Autodesk Inventor part; units mm, degrees
ref_plane "YZ Plane" through (0, 0, 0) normal (1, 0, 0) x (0, 1, 0)
ref_plane "XZ Plane" through (0, 0, 0) normal (0, 1, 0) x (-1, 0, 0)
ref_plane "XY Plane" through (0, 0, 0) normal (0, 0, 1) x (1, 0, 0)
sketch "Sketch1" plane through (0, 0, 0) normal (0, 0, 1) x (1, 0, 0)
  line L0 (-15.9912, -11.7475) -> (15.7588, -11.7475)
  line L1 (15.7588, -11.7475) -> (15.7588, 14.2875)
  line L2 (-15.9912, 14.2875) -> (-15.9912, -11.7475)
  line L3 (-15.9912, -11.7475) -> (15.7588, 11.5768) construction
  line L4 (15.7588, -11.7475) -> (-15.9912, 11.9207) construction
  line L5 (19.1662, -14.2875) -> (-19.1662, -14.2875)
  line L6 (-19.1662, -14.2875) -> (-19.1662, 14.2875)
  line L7 (19.1662, 14.2875) -> (19.1662, -14.2875)
  line L8 (19.1662, -14.2875) -> (-19.1662, 14.2875) construction
  line L9 (-19.1662, -14.2875) -> (19.1662, 14.2875) construction
  line L10 (-19.1662, 14.2875) -> (-15.9912, 14.2875)
  line L11 (15.7588, 14.2875) -> (19.1662, 14.2875)
  point P0 (0, 0)
  dimension "d2" = 3.175
  dimension "d3" = 28.575
  dimension "d4" = 31.75
  dimension "d5" = 2.54
extrude "Extrusion1" add sketch "Sketch1" along normal mid plane 25.4
sketch "Sketch2" plane through (19.1662, 14.2875, 12.7) normal (1, 0, 0) x (0, 0, -1)
  line L0 (0, 0) -> (25.4, 0)
  point P0 (12.7, -14.2875)
  point P1 (12.7, -12.7)
  dimension "d9" = 12.7
hole "Hole1" at (19.1662, 1.5875, 0) direction (-1, 0, 0) diameter 6.7564 end through all
sketch "Sketch3" plane through (-15.9912, -11.7475, 12.7) normal (0, 1, 0) x (1, 0, 0)
  line L0 (0, 25.4) -> (0, 0)
  line L1 (0, 25.4) -> (31.75, 25.4)
  point P0 (15.875, 12.7)
  point P1 (15.875, 12.7)
  dimension "d26" = 12.7
  dimension "d27" = 15.875
hole "Hole2" at (-0.1162, -11.7475, 0) direction (0, -1, 0) diameter 6.7564 end through all
fillet "Fillet2" radius 3.175 2 edges at (-19.1662, -14.2875, 0) (19.1662, -14.2875, 0)
fillet "Fillet3" radius 1.5875 2 edges at (-15.9912, -11.7475, 0) (15.7588, -11.7475, 0)
sketch "Sketch4" plane through (-19.1662, 14.2875, -12.7) normal (-1, 0, 0) x (0, 0, 1)
  circle A0 centre (12.7, -12.7) radius 3.3782
  circle A1 centre (12.7, -12.7) radius 728.218
  line L0 (723.9, -1.1049) -> (723.9, 7.4549)
  circle A2 centre (653.833, 332.6257) radius 3.5687
  point P0 (12.7, -14.2875)
  point P1 (723.9, 143.812)
properties part number "C19_TK_ClimberingSupportBracket" material "Aluminum 6061"
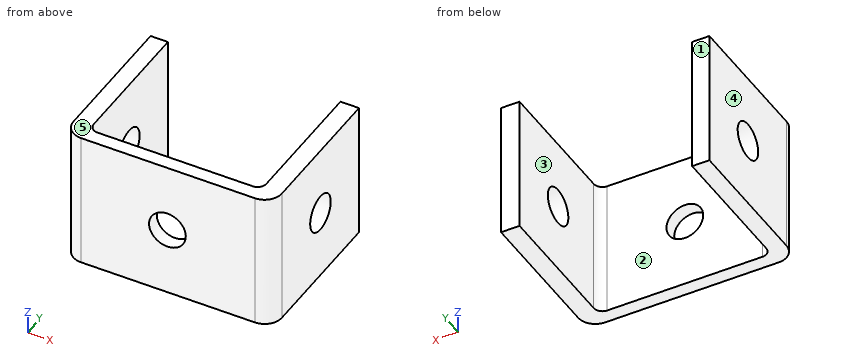
Build history of the part. All positions in model axes, mm. Face numbers are marked on the shaded views. A direction names the side the tool comes from. Coordinates: 2 decimals unless noted, no trailing zeros. Order: outer loops, then holes, each group sorted by start corner. A loop starts at its lowest first (then second) coordinate and runs counter-clockwise, first axis right, second up. Notation, with made-up numbers: (-1, 45) - (52, 45) arc R11 ccw to (52, 53) - close; hole circle Ø8 at (-13, 34.5). An arc over 180 degrees is marked (long way). Write item = value, one per line. Start each with the question number.
1) Wall check: line 1 along X through (y, z) = (4.25, -9); line 2 along Y through (x, z) = (-5.5, 6); line 3 along Y through (x, z) = (-18, 0). Give the ranges that are in metal, low to high. Write a range as from..to.
2) Flat gauge pins, fed straight in: pin 1 Ø6 at (y, z) = (1.59, 0) entering from +X; pin 2 Ø5 at (x, z) = (-11, 8.5) entering from +Y. Where does each tip first touch, or does it go through?
3) Saw through at B-B on y = -9. Write the cut outline in (x, z), then the cut area to 3 significant figures.
4) 3-axis set-ups, long thin cutter, end or side, ignore diameter. For the marked faces 1 and 2: which of +Z, -Z, +X, -X, +Y, -Y reach the whole face in a straight line?
5) Saw through at A-A on z = 0. Count the separate pieces of the cut face and the enclosed holes in it, then the cut area to 3 significant figures.
6) Two-plate mould, pull along X, no slides. Class the marked faces 3, 4 and 5: pulls with the +X half, pulls with the -X half, needs draft (parallel to the pull), parting line crosses it, or undercut.
7) Saw through at D-D on y = -0.5. Write the cut outline in (x, z).
From the geometry:
q1.line_1 = -19.17..-15.99, 15.76..19.17
q1.line_2 = -14.29..-11.75
q1.line_3 = -13.57..-1.79, 4.97..14.29
q2.pin_1 = through
q2.pin_2 = -11.75
q3.outline = (-19.17, -12.7) - (-15.99, -12.7) - (-15.99, 12.7) - (-19.17, 12.7) - close; (15.76, -12.7) - (19.17, -12.7) - (19.17, 12.7) - (15.76, 12.7) - close
q3.area = 167 mm^2
q4.face_1 = +Z, -Z, +X, -X, +Y
q4.face_2 = +Z, -Z, +Y
q5.separate_pieces = 4
q5.enclosed_holes = 0
q5.area = 204 mm^2
q6.face_3 = undercut
q6.face_4 = pulls with the -X half
q6.face_5 = needs draft
q7.outline = (-19.17, -12.7) - (-15.99, -12.7) - (-15.99, -2.66) - (-19.17, -2.66) - close; (-19.17, 2.66) - (-15.99, 2.66) - (-15.99, 12.7) - (-19.17, 12.7) - close; (15.76, -12.7) - (19.17, -12.7) - (19.17, -2.66) - (15.76, -2.66) - close; (15.76, 2.66) - (19.17, 2.66) - (19.17, 12.7) - (15.76, 12.7) - close
